Autodesk Inventor part; units mm, degrees
ref_plane "YZ Plane" through (0, 0, 0) normal (1, 0, 0) x (0, 1, 0)
ref_plane "XZ Plane" through (0, 0, 0) normal (0, 1, 0) x (-1, 0, 0)
ref_plane "XY Plane" through (0, 0, 0) normal (0, 0, 1) x (1, 0, 0)
sketch "Sketch1" plane through (0, 0, 0) normal (0, 1, 0) x (-1, 0, 0)
  circle A0 centre (0, 0) radius 11
  dimension "d0" = 22
extrude "Extrusion1" add sketch "Sketch1" along normal blind 25
sketch "Sketch2" plane through (0, 0, 0) normal (0, -1, 0) x (1, 0, 0)
  circle A0 centre (0, 0) radius 9.5
  dimension "d3" = 19
extrude "Extrusion2" cut sketch "Sketch2" against normal blind 10
sketch "Sketch3" plane through (0, 25, 0) normal (0, 1, 0) x (1, 0, 0)
  circle A0 centre (0, 0) radius 8.98
  dimension "d6" = 17.96
extrude "Extrusion3" cut sketch "Sketch3" against normal blind 13
chamfer "Chamfer1" distance 2 angle 45 1 edges at (-8.98, 25, 0) measured on face at (-10.1331, 25, -1.5938)
properties part number "Cup"
Design review of the part built by this model. Coordinates are the model's own, in mm. A direction names the side the tool comes from. Round coordinates to 2 decimals unless told otherwise and drop trailing zeros. Loops run counter-clockwise (first coordinate to the right, second up) from the corner with the lowest first, then second, coordinate; pieces in that order, holes last. Notation, with made-up numbers: M 6,0 L 61,0 A14 ccw 61,22 Z; hole C -7,75.25 d5. An arc over 180 degrees is marked long. Answer as a JSON object with one key per item and string values.
Item 1: The part is to be moulded in two halves that separate along Z. For faces 3 (the cylindrical face through (2.38, 12.32, 10.74)), 4 (the conical face through (-1.974, 23.125, 8.889)), 5 (the cylindrical face through (4.38, 4.93, -8.43)), 6 (the flat face through (10, 0, 0)), say which applies: pulls with the +Z half, pulls with the -Z half, needs draft (parallel to the pull), parting line crosses it, or undercut.
Answer sheet:
{"face 3": "parting line crosses it", "face 4": "undercut", "face 5": "undercut", "face 6": "needs draft"}
Item 2: Wall thickness on L1, parallel to Z at x = 0, y = 16.25; L2, parallel to Y at x = -8.5, z = 2.25; L3, parallel to X at y = 20.75, z = 6: over which ranges is each line inside the solid? List them lowest first. Write a range as from..to.
Answer sheet:
{"L1": "z = -11..-8.98, 8.98..11", "L2": "y = 10..12", "L3": "x = -9.22..-6.68, 6.68..9.22"}
Item 3: Clearance check with flat-ended pins moving along their axes: P1, Ø2, axis at x = -4, y = 12, coming from the -Z side; P2, Ø2, axis at x = -2.5, z = -7, coming from the -Y side; P3, Ø12, axis at x = 3, y = 11.5, coming from the +Z side; P4, Ø5, axis at y = 10, z = -6, coming from the -X side. State where each tip first meets the part, or that it passes through.
Answer sheet:
{"P1": "stops at z = -10.58", "P2": "stops at y = 10", "P3": "stops at z = 11", "P4": "stops at x = -10.43"}
Item 4: We need section D-D on y = 10.75. Give the boundary of the cut face in (x, z).
Answer sheet:
{"outline": "C 0,0 d22"}
Item 5: Machinability: for faces 1 (the flat face through (0, 10, 0)), 2 (the flat face through (0, 12, 0)), which of the approach directions +Z, -Z, +X, -X, +Y, -Y give a long, thin tool a straight path to every point of the face, cutting with its end or side? Answer none if there is none.
Answer sheet:
{"face 1": "-Y", "face 2": "+Y"}
Item 6: We need section C-C on y = 17.5. Give the boundary of the cut face in (x, z).
Answer sheet:
{"outline": "C 0,0 d22; hole C 0,0 d17.96"}
